from build123d import *

# Parameters (mm, degrees)
SKETCH_1_W      = 117.11
SKETCH_1_H      = 112.14
EXTRUDE_1_DEPTH = 33.65
SKETCH_2_R      = 5
EXTRUDE_2_DEPTH = 3
FILLET_1_R      = 2


with BuildPart() as part:
    # 草图1 → 凸台-拉伸1 (new body)
    with BuildSketch(Plane(origin=(0, 0, 0), x_dir=(1, 0, 0), z_dir=(0, 1, 0))):
        Rectangle(SKETCH_1_W, SKETCH_1_H)
    extrude(amount=EXTRUDE_1_DEPTH)

    # 草图2 → 凸台-拉伸2 (add)
    with BuildSketch(Plane.XZ):
        with Locations((-47, 46)):
            Circle(SKETCH_2_R)
        with Locations((47, 46)):
            Circle(SKETCH_2_R)
        with Locations((47, -46)):
            Circle(SKETCH_2_R)
        with Locations((-47, -46)):
            Circle(SKETCH_2_R)
    extrude(amount=EXTRUDE_2_DEPTH)

    # 圆角1
    fillet_1_edges = [part.edges().sort_by_distance(p)[0] for p in [
        (-58.555, 33.65, 0),
        (0, 33.65, 56.07),
        (58.555, 33.65, 0),
        (58.555, 16.825, 56.07),
        (-58.555, 16.825, 56.07),
        (-58.555, 16.825, -56.07),
        (58.555, 16.825, -56.07),
        (0, 33.65, -56.07),
    ]]
    fillet(fillet_1_edges, radius=FILLET_1_R)


solid = part.part
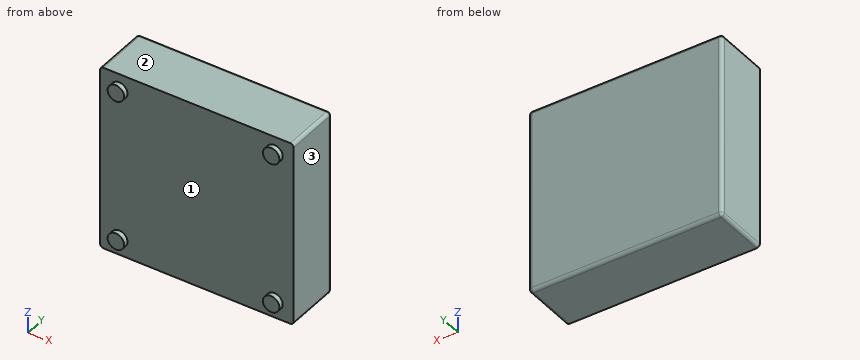
Work out the finished part from the listing and answer in its coordinate system (mm). Face numbers are marked on the shaded views. Give positions to 0.01 mm unless a question says otherwise; leave off trailing zeros. Write each loop counter-clockwise with the first axis right and the second up, starting at its lowest first coordinate (ties: lowest second). Pieces come first, ordered by that corner, then holes.
Q1. Given pin 1 (3 mm diameter, centred on x = 21, z = 23.5, fed in from -Y), flat-ended and moving along its own axis, determine where the tip first touches the part or whether it passes through.
Answer:
pin 1: stops at y = 0
Q2. Straight lines are drawn through the part: L1, parallel to Y at x = -3, z = 39; L2, parallel to Z at x = -36, y = 32.5. For each, find the intervals that lie inside material, in ascending order.
Answer:
L1: y = 0 to 33.65
L2: z = -55.88 to 55.88
Q3. The part is cut by section C-C on z = -5.5. Give the vertices of the cut face in (x, y) (3 decimals).
Answer:
outline: (-58.555, 0) - (58.555, 0) - (58.555, 31.65) arc R2 ccw to (56.555, 33.65) - (-56.555, 33.65) arc R2 ccw to (-58.555, 31.65) - close
Q4. The part is cut by section A-A on z = 46. Give the vertices of the cut face in (x, y) (3 decimals).
Answer:
outline: (-58.555, 0) - (-52, 0) - (-52, -3) - (-42, -3) - (-42, 0) - (42, 0) - (42, -3) - (52, -3) - (52, 0) - (58.555, 0) - (58.555, 31.65) arc R2 ccw to (56.555, 33.65) - (-56.555, 33.65) arc R2 ccw to (-58.555, 31.65) - close
Q5. The part is cut by section B-B on x = 47. Give the vertices of the cut face in (y, z).
Answer:
outline: (-3, -51) - (0, -51) - (0, -56.07) - (31.65, -56.07) arc R2 ccw to (33.65, -54.07) - (33.65, 54.07) arc R2 ccw to (31.65, 56.07) - (0, 56.07) - (0, 51) - (-3, 51) - (-3, 41) - (0, 41) - (0, -41) - (-3, -41) - close
Q6. The part is cut by section D-D on x = 31. Give the vertices of the cut face in (y, z).
Answer:
outline: (0, -56.07) - (31.65, -56.07) arc R2 ccw to (33.65, -54.07) - (33.65, 54.07) arc R2 ccw to (31.65, 56.07) - (0, 56.07) - close
Q7. For a pull along X with two mould halves and no side action, classify the marked faces 1, 2 and 3 as released by +X, released by -X, zero draft, split by the parting line, or undercut.
Answer:
face 1: undercut
face 2: zero draft
face 3: released by +X
